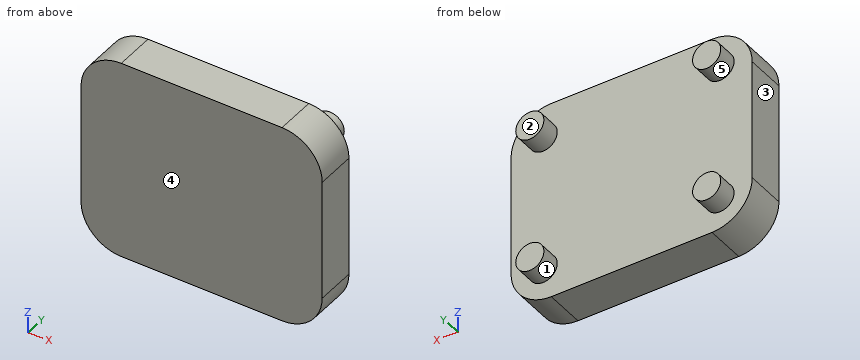
```python
from build123d import *

# Parameters (mm, degrees)
BOSS_EXTRUDE1_DEPTH = 2
SKETCH3_R           = 0.7
BOSS_EXTRUDE3_DEPTH = 1


with BuildPart() as part:
    # Sketch1 → Boss-Extrude1 (new body)
    with BuildSketch(Plane(origin=(0, 0, 0), x_dir=(1, 0, 0), z_dir=(0, 1, 0))):
        with BuildLine():
            Line((-2, 0), (-10, 0))
            ThreePointArc((-10, 0), (-11.414213562, -0.585786438), (-12, -2))
            Line((-12, -2), (-12, -8))
            ThreePointArc((-12, -8), (-11.414213562, -9.414213562), (-10, -10))
            Line((-10, -10), (-2, -10))
            ThreePointArc((-2, -10), (-0.585786438, -9.414213562), (0, -8))
            Line((0, -8), (0, -2))
            ThreePointArc((0, -2), (-0.585786438, -0.585786438), (-2, 0))
        make_face()
    extrude(amount=BOSS_EXTRUDE1_DEPTH)

    # Sketch3 → Boss-Extrude3 (add)
    with BuildSketch(Plane(origin=(0, 2, 0), x_dir=(1, 0, 0), z_dir=(0, 1, 0))):
        with Locations(Location((-10.4, -1.6, 0), (0, 0, 90))):
            Circle(SKETCH3_R)
        with Locations(Location((-1.6, -1.6, 0), (0, 0, 90))):
            Circle(SKETCH3_R)
        with Locations(Location((-1.6, -8.4, 0), (0, 0, 90))):
            Circle(SKETCH3_R)
        with Locations(Location((-10.4, -8.4, 0), (0, 0, 90))):
            Circle(SKETCH3_R)
    extrude(amount=BOSS_EXTRUDE3_DEPTH)


solid = part.part
```
The listing builds one solid part. Answer for the finished solid, in the listing's coordinates (mm). Face numbers are marked on the shaded views. A direction names the side the tool comes from. Give positions to 0.01 mm unless a question says otherwise; leave off trailing zeros. Write each loop counter-clockwise with the first axis right and the second up, starting at its lowest first coordinate (ties: lowest second). Pieces come first, ordered by that corner, then holes. Notation, with made-up numbers: (18, 60) -> (27, 60) arc R25 ccw to (27, 98) -> close; hole circle Ø8 at (48.5, 17). An arc over 180 degrees is marked (long way). Write item = value, one per line. Start each with the question number.
1) Which of the six approach directions +Z, -Z, +X, -X, +Y, -Y give full straight-line access (tool end or side, diameter ignored) to the marked faces 1 and 2?
2) Determine the mould class of the marked faces 3, 4 and 5 for opening direction X: +X half, -X half, draft (parallel to the pull), parting line (faces both ways), or undercut.
3) The part is cut by section A-A, the plane y = 0.3. Determine the outline of the cut face in (x, z), and give its area (3 significant figures).
4) The part is cut by section B-B, the plane y = 2.6. Determine the outline of the cut face in (x, z), and give its area (3 significant figures).
5) This flat-tipped pin is pushed along its axis until it touches: pin 1 (1.5 mm diameter, centred on y = 1.5, z = 9, fed in from +X). Where does it stop, or does it pass through?
6) The part is cut by section D-D, the plane x = -10.4. Determine the outline of the cut face in (y, z), and give its area (3 significant figures).
7) The part is cut by section C-C, the plane z = 1.6. Determine the outline of the cut face in (x, y).
8) Straight lines are drawn through the part: line 1 along Y through (x, z) = (-5.5, 3); line 2 along X through (y, z) = (2.35, 8.5); line 3 along X through (y, z) = (0.8, 8.25). For each, find the intervals that lie inside material, in ascending order.
Solutions:
q1.face_1 = +Y
q1.face_2 = +Z, -Z, +X, -X, +Y
q2.face_3 = -X half
q2.face_4 = draft
q2.face_5 = undercut
q3.outline = (-12, 2) arc R2 ccw to (-10, 0) -> (-2, 0) arc R2 ccw to (0, 2) -> (0, 8) arc R2 ccw to (-2, 10) -> (-10, 10) arc R2 ccw to (-12, 8) -> close
q3.area = 117 mm²
q4.outline = circle Ø1.4 at (-10.4, 1.6); circle Ø1.4 at (-10.4, 8.4); circle Ø1.4 at (-1.6, 1.6); circle Ø1.4 at (-1.6, 8.4)
q4.area = 6.16 mm²
q5.pin_1 = -0.02
q6.outline = (0, 0.04) -> (2, 0.04) -> (2, 0.9) -> (3, 0.9) -> (3, 2.3) -> (2, 2.3) -> (2, 7.7) -> (3, 7.7) -> (3, 9.1) -> (2, 9.1) -> (2, 9.96) -> (0, 9.96) -> close
q6.area = 22.6 mm²
q7.outline = (-11.96, 0) -> (-0.04, 0) -> (-0.04, 2) -> (-0.9, 2) -> (-0.9, 3) -> (-2.3, 3) -> (-2.3, 2) -> (-9.7, 2) -> (-9.7, 3) -> (-11.1, 3) -> (-11.1, 2) -> (-11.96, 2) -> close
q8.line_1 = 0 to 2
q8.line_2 = -11.09 to -9.71, -2.29 to -0.91
q8.line_3 = -11.98 to -0.02
